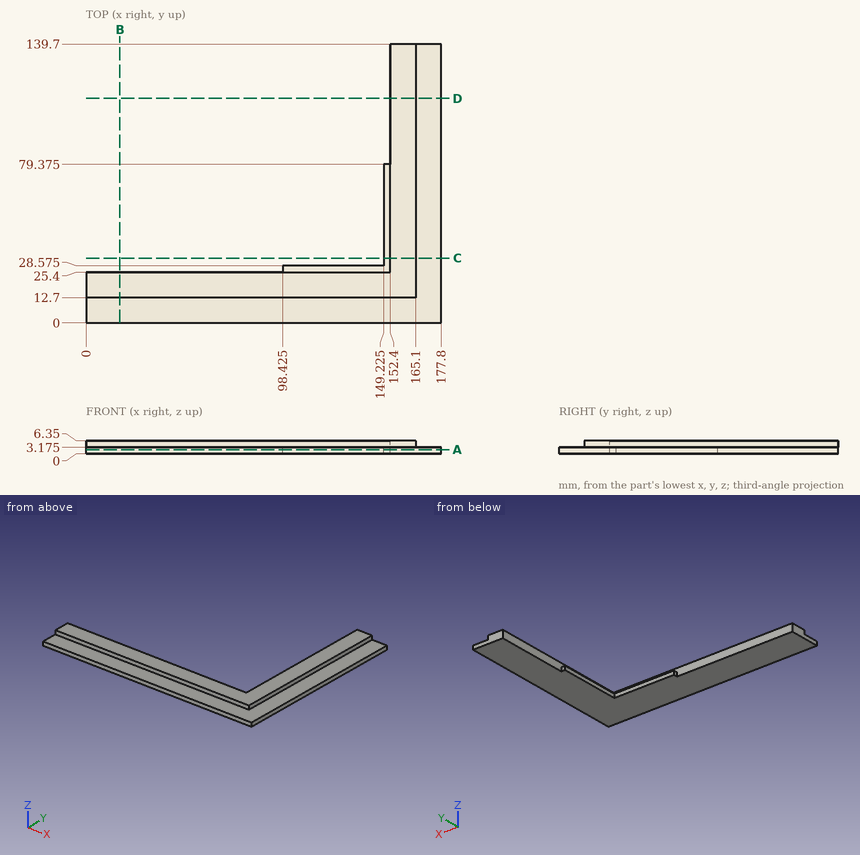
Geometry check sheet. Reference: drawing and pictorial views, mm from the part's lowest x, y, z. Round coordinates to 2 decimals unless told otherwise and drop trailing zeros. Write each loop counter-clockwise with the first axis right and the second up, starting at its lowest first coordinate (ties: lowest second). Pieces come first, ordered by that corner, then holes. Notation, with made-up numbers: (-28.5, 78) -> (28.5, 78) arc R17 ccw to (28.5, 95) -> close; hole circle Ø1 at (-3.75, 72.5). An arc over 180 degrees is marked (long way). Put each result on its own line as item: value.
1) Depth check by flat-ended pin: P1, Ø3, axis at y = 71.5, z = 4, coming from the -X side (3 decimals); P2, Ø1.6, axis at y = 27, z = 1.5, coming from the -X side (3 decimals); P3, Ø3.5, axis at x = 82, z = 5, coming from the -Y side; P4, Ø6, axis at x = 66.5, y = 26, coming from the -Z side. Enter the tip coordinate at first touch or a pass-through.
Recorded:
P1: stops at x = 149.225
P2: stops at x = 98.425
P3: stops at y = 12.7
P4: stops at z = 0
2) Cross-section at B-B, the plane x = 17. Enter the section's corners in (y, z) (3 decimals), plus the area to 3 significant figures.
Recorded:
outline: (0, 0) -> (25.4, 0) -> (25.4, 6.35) -> (12.7, 6.35) -> (12.7, 3.175) -> (0, 3.175) -> close
area: 121 mm2
3) Cross-section at D-D, the plane y = 112.5. Enter the section's corners in (x, z) (3 decimals).
Recorded:
outline: (152.4, 0) -> (177.8, 0) -> (177.8, 3.175) -> (165.1, 3.175) -> (165.1, 6.35) -> (152.4, 6.35) -> close
4) Cross-section at C-C, the plane y = 32.5. Enter the section's corners in (x, z) (3 decimals).
Recorded:
outline: (149.225, 0) -> (177.8, 0) -> (177.8, 3.175) -> (165.1, 3.175) -> (165.1, 6.35) -> (152.4, 6.35) -> (152.4, 3.175) -> (149.225, 3.175) -> close
5) Thickness scan on probe 1 along Y at (x, z) = (61, 4.25); probe 2 along Y at (x, z) = (52, 1.5); probe 3 along X at (y, z) = (20, 5.75). Record the ranges inside material, lowest first. Write a range as from..to.
Recorded:
probe 1: y = 12.7..25.4
probe 2: y = 0..25.4
probe 3: x = 0..165.1
6) Cross-section at A-A, the plane z = 2. Enter the section's corners in (x, y) (3 decimals).
Recorded:
outline: (0, 0) -> (177.8, 0) -> (177.8, 139.7) -> (152.4, 139.7) -> (152.4, 79.375) -> (149.225, 79.375) -> (149.225, 28.575) -> (98.425, 28.575) -> (98.425, 25.4) -> (0, 25.4) -> close
